The drawing under review shows one solid part. Ordinate dimensions are in mm from its lowest x, y, z. A direction names the side the tool comes from. Give positions to 0.01 mm unless a question says otherwise; leave off trailing zeros. Loops run counter-clockwise (first coordinate to the right, second up) from the corner with the lowest first, then second, coordinate; pieces in that order, holes last. Notation, with made-up numbers: (-10.75, -29.5) - (25.25, -29.5) arc R15 ccw to (25.25, -3.5) - close; hole circle Ø4 at (8, 44). An arc over 180 degrees is marked (long way). Return JSON: item names as keys, results as strings. Group by question number.
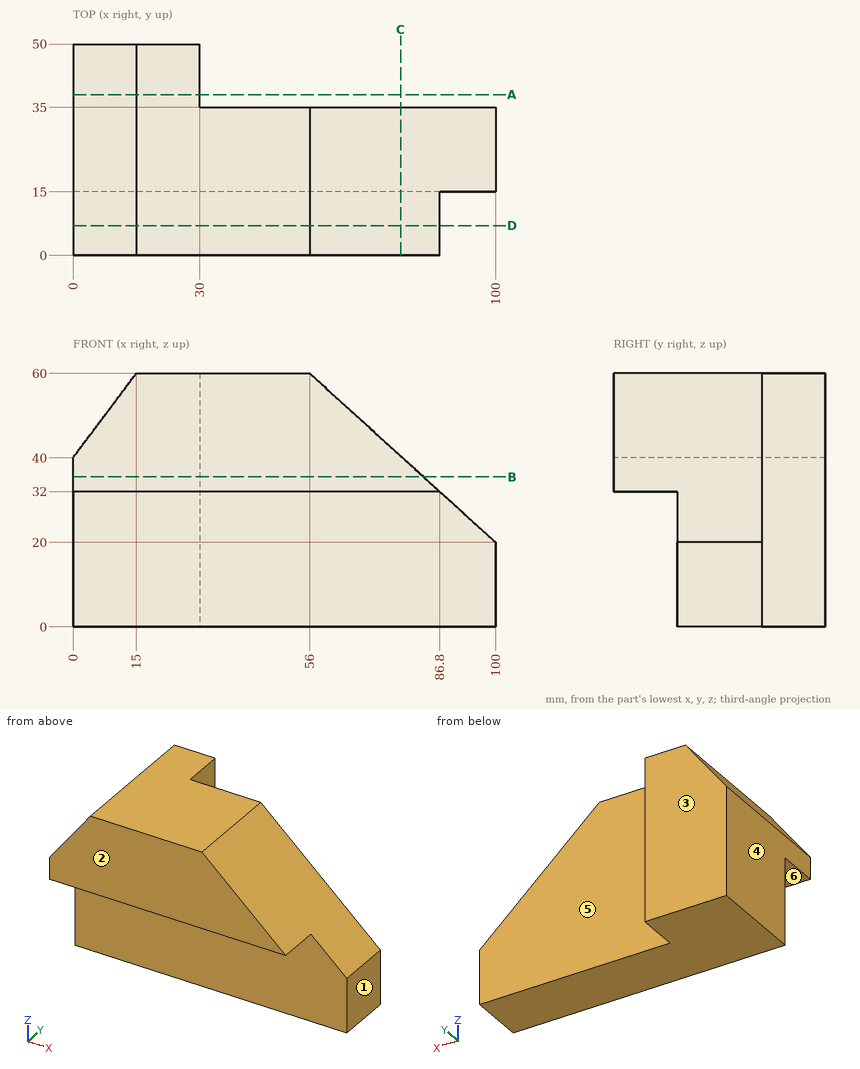
1) We need section A-A, the plane y = 38. Write out the cut boundary in (x, z), plus the area to 3 significant figures.
2) Tool access review of the marked faces 4, 5 and 6: name each direction out of +Z, -Z, +X, -X, +Y, -Y from which nothing blocks a thin tool from reaching the whole face with its end or side.
3) We need section B-B, the plane z = 35.5. Write out the cut boundary in (x, y), plus the area to 3 significant figures.
4) We need section D-D, the plane y = 7. Write out the cut boundary in (x, z).
5) To check wall thickness, follow line 1 (Y direction, x = 90.5, z = 4.5); line 2 (Z direction, x = 28, y = 2); line 3 (X direction, y = 38, z = 11.5). State the ranges of each line that lie inside material, in increasing order.
6) For pin 1 Ø16.5 at (x, y) = (22, 5.5) entering from -Z; pin 2 Ø2 at (x, z) = (14, 9.5) entering from -Y; pin 3 Ø8 at (y, z) = (31.5, 22.5) entering from +X; pin 4 Ø8 at (x, y) = (83.5, 29.5) entering from +Z, all flat-tipped, find the tip position at first contact; note any pin that passes through.
7) We need section C-C, the plane x = 77.5. Write out the cut boundary in (y, z), plus the area to 3 significant figures.
8) Draft analysis for pull direction Y (two halves, no side actions). For the marked faces 1, 2 and 3, state which applies: +Y half, -Y half, draft (parallel to the pull), parting line (faces both ways), or undercut.
Findings:
{
 "1": {"outline": "(0, 0) - (30, 0) - (30, 60) - (15, 60) - (0, 40) - close", "area": "1,650 mm^2"},
 "2": {"face 4": "+Z, -Z, -X, +Y, -Y", "face 5": "+Z, -Z, +X, +Y", "face 6": "-Z, +X, -X, -Y"},
 "3": {"outline": "(0, 0) - (82.95, 0) - (82.95, 35) - (30, 35) - (30, 50) - (0, 50) - close", "area": "3,350 mm^2"},
 "4": {"outline": "(0, 32) - (86.8, 32) - (56, 60) - (15, 60) - (0, 40) - close"},
 "5": {"line 1": "y = 15 to 35", "line 2": "z = 32 to 60", "line 3": "x = 0 to 30"},
 "6": {"pin 1": "stops at z = 32", "pin 2": "stops at y = 15", "pin 3": "stops at x = 100", "pin 4": "stops at z = 38.64"},
 "7": {"outline": "(0, 32) - (15, 32) - (15, 0) - (35, 0) - (35, 40.45) - (0, 40.45) - close", "area": "936 mm^2"},
 "8": {"face 1": "draft", "face 2": "-Y half", "face 3": "+Y half"}
}
